Source: CAD feature listing. Evaluate the final solid. Frame: model axes, mm. Round coordinates to 2 decimals unless told otherwise and drop trailing zeros. Write each loop counter-clockwise with the first axis right and the second up, starting at its lowest first coordinate (ties: lowest second). Pieces come first, ordered by that corner, then holes. Notation, with made-up numbers: M -23,88.25 L 34,88.25 A25 ccw 34,120.25 Z; hole C -12.75,56.5 d9. An arc over 180 degrees is marked long. Answer in a Markdown table with one row per item.
from build123d import *

# Parameters (mm, degrees)
F0_R     = 2
F0_R_2   = 1
F1_DEPTH = 1.2


with BuildPart() as f1:
    # F0 (on Top) → F1 (new body)
    with BuildSketch(Plane.XY):
        Polygon((-41.936022, 88.209298), (-54.636022, 88.209298), (-54.636022, 19.629298), (-41.936022, 19.629298), (-41.936022, 75.509298), (-16.536022, 75.509298), (-16.536022, 19.629298), (-3.836022, 19.629298), (-3.836022, 88.209298), (-16.536022, 88.209298), align=None)
        with Locations((-49.556022, 24.709298)):
            Circle(F0_R, mode=Mode.SUBTRACT)
        with Locations((-49.556022, 31.059298)):
            Circle(F0_R, mode=Mode.SUBTRACT)
        with Locations((-7.011022, 22.804298)):
            Circle(F0_R_2, mode=Mode.SUBTRACT)
        with Locations((-7.011022, 37.804298)):
            Circle(F0_R_2, mode=Mode.SUBTRACT)
    extrude(amount=F1_DEPTH)


solid = f1.part
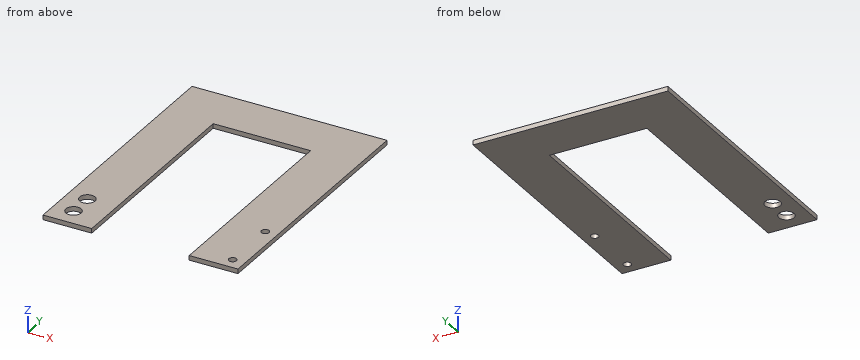
Q1. Section A-A (y = 64.5). Return loops of the section in (x, z).
Solutions:
| item | result |
|---|---|
| outline | M -54.64,0 L -41.94,0 L -41.94,1.2 L -54.64,1.2 Z; M -16.54,0 L -3.84,0 L -3.84,1.2 L -16.54,1.2 Z |
Q2. Section C-C (x = -20.5). Return loops of the section in (y, z).
Solutions:
| item | result |
|---|---|
| outline | M 75.51,0 L 88.21,0 L 88.21,1.2 L 75.51,1.2 Z |
Q3. Material intervals for probe 1 along Y at (x, z) = (-49.5, 0.7); probe 2 along X at (y, z) = (50.5, 0.65); probe 3 along X at (y, z) = (26.5, 0.15), sorted ascending.
Solutions:
| item | result |
|---|---|
| probe 1 | y = 19.63 to 22.71, 26.71 to 29.06, 33.06 to 88.21 |
| probe 2 | x = -54.64 to -41.94, -16.54 to -3.84 |
| probe 3 | x = -54.64 to -50.45, -48.67 to -41.94, -16.54 to -3.84 |
Q4. Section B-B (z = 0.55). Return loops of the section in (x, y), and give its area (3 significant figures).
Solutions:
| item | result |
|---|---|
| outline | M -54.64,19.63 L -41.94,19.63 L -41.94,75.51 L -16.54,75.51 L -16.54,19.63 L -3.84,19.63 L -3.84,88.21 L -54.64,88.21 Z; hole C -49.56,24.71 d4; hole C -49.56,31.06 d4; hole C -7.01,22.8 d2; hole C -7.01,37.8 d2 |
| area | 2,030 mm2 |
